Autodesk Inventor part; units mm, degrees
ref_plane "YZ Plane" through (0, 0, 0) normal (1, 0, 0) x (0, 1, 0)
ref_plane "XZ Plane" through (0, 0, 0) normal (0, 1, 0) x (-1, 0, 0)
ref_plane "XY Plane" through (0, 0, 0) normal (0, 0, 1) x (1, 0, 0)
sketch "Sketch1" plane through (0, 0, 0) normal (0, 1, 0) x (-1, 0, 0)
  line L0 (-7.5, 17.5) -> (7.5, 17.5) construction
  line L1 (7.5, 17.5) -> (7.5, -17.5)
  line L2 (7.5, -17.5) -> (-7.5, -17.5) construction
  line L3 (-7.5, -17.5) -> (-7.5, 17.5)
  line L4 (-7.5, 17.5) -> (7.5, -17.5) construction
  line L5 (7.5, 17.5) -> (-7.5, -17.5) construction
  circle A0 centre (0, 17.5) radius 2.5
  circle A1 centre (0, 17.5) radius 7.5
  circle A2 centre (0, -17.5) radius 2.5
  circle A3 centre (0, -17.5) radius 7.5
  point P0 (0, 0)
  point P1 (-7.5, 17.5)
  point P2 (-7.5, -17.5)
  dimension "d4" = 15
  dimension "d0" = 35
  dimension "d1" = 15
  dimension "d5" = 5
  dimension "d6" = 5
extrude "Extrusion1" add sketch "Sketch1" along normal blind 5
equation "\"d4\" = d1"
equation "\"d6\" = d5"
properties part number "scissor-link"
Part model, mm, in its own coordinate system. Give positions to 0.01 mm unless a question says otherwise; leave off trailing zeros. Loops run counter-clockwise (first coordinate to the right, second up) from the corner with the lowest first, then second, coordinate; pieces in that order, holes last. Notation, with made-up numbers: M 18.25,29 L 33.25,29 A15 cw 33.25,34 Z; hole C 84.5,-4.5 d3. An arc over 180 degrees is marked long. Put each result on its own line as item: value. Start each with the question number.
1) Saw through at D-D (z = 19). List the corners of the cut face in (x, y), then the cut area to 3 significant figures.
2) Saw through at B-B (z = -15.5). List the corners of the cut face in (x, y), then the cut area to 3 significant figures.
3) Saw through at C-C (y = 0.5). List the corners of the cut face in (x, z), then the cut area to 3 significant figures.
4) Pull direction Z, two halves, no side cores. Call faces 1 (the cylindrical face through (0, 2, -25)), 2 (the cylindrical face through (0, 2, 25)), 3 (the cylindrical face through (0.54, 2.46, 19.94)), 4 (the flat face through (0, 5, 0)): +Z half, -Z half, draft (parallel to the pull), parting line (faces both ways), or undercut.
5) Probe probe 1 along Z at (x, y) = (0, 3.45); probe 2 along Z at (x, y) = (-1, 3.7); probe 3 along X at (y, z) = (3.9, -18.5). List the from-to ranges inside material, lowest first.
6) Flat gauge pin, fed straight in: pin 1 (2 mm diameter, centred on x = 2.5, y = 1.5, fed in from -Z). Where does the tip first touch, or does it go through?
7) Saw through at A-A (x = 0). List the corners of the cut face in (y, z).
Numbers:
1. outline: M -7.35,0 L -2,0 L -2,5 L -7.35,5 Z; M 2,0 L 7.35,0 L 7.35,5 L 2,5 Z
1. area: 53.5 mm^2
2. outline: M -7.5,0 L -1.5,0 L -1.5,5 L -7.5,5 Z; M 1.5,0 L 7.5,0 L 7.5,5 L 1.5,5 Z
2. area: 60.0 mm^2
3. outline: M -7.5,-17.5 A7.5 ccw 7.5,-17.5 L 7.5,17.5 A7.5 ccw -7.5,17.5 Z; hole C 0,-17.5 d5; hole C 0,17.5 d5
3. area: 662 mm^2
4. face 1: -Z half
4. face 2: +Z half
4. face 3: undercut
4. face 4: draft
5. probe 1: -25 to -20, -15 to 15, 20 to 25
5. probe 2: -24.93 to -19.79, -15.21 to 15.21, 19.79 to 24.93
5. probe 3: -7.43 to -2.29, 2.29 to 7.43
6. pin 1: z = -24.85
7. outline: M 0,-25 L 5,-25 L 5,-20 L 0,-20 Z; M 0,-15 L 5,-15 L 5,15 L 0,15 Z; M 0,20 L 5,20 L 5,25 L 0,25 Z
